from build123d import *

# Parameters (mm, degrees)
F0_R     = 35
F1_DEPTH = 6.5
F2_R     = 23.5
F3_DEPTH = 6.5
F4_R     = 32
F4_R_2   = 26
F5_DEPTH = 4
F7_DEPTH = 2
F8_R     = 6
F9_DEPTH = 4


with BuildPart() as f1:
    # F0 (on Top) → F1 (new body)
    with BuildSketch(Plane.XY):
        Circle(F0_R)
    extrude(amount=F1_DEPTH)

    # F2 (on face) → F3 (cut, through all)
    with BuildSketch(Plane.XY.offset(6.5)):
        Circle(F2_R)
    extrude(amount=-F3_DEPTH, mode=Mode.SUBTRACT)

    # F4 (on face) → F5 (cut)
    with BuildSketch(Plane(origin=(0, 0, 0), x_dir=(1, 0, 0), z_dir=(0, 0, -1))):
        Circle(F4_R)
        Circle(F4_R_2, mode=Mode.SUBTRACT)
    extrude(amount=-F5_DEPTH, mode=Mode.SUBTRACT)

    # F6 (on Top) → F7 (cut)
    with BuildSketch(Plane.XY):
        Polygon((-26, 5), (-26, -5), (-8.6602540378, -5), (-17.3301270189, -20.0166604984), (-8.6698729811, -25.0166604984), (0, -10), (8.6698729811, -25.0166604984), (17.3301270189, -20.0166604984), (8.6602540378, -5), (26, -5), (26, 5), (8.6602540378, 5), (17.3301270189, 20.0166604984), (8.6698729811, 25.0166604984), (0, 10), (-8.6698729811, 25.0166604984), (-17.3301270189, 20.0166604984), (-8.6602540378, 5), align=None)
    extrude(amount=F7_DEPTH, mode=Mode.SUBTRACT)

    # F8 (on Top) → F9 (join)
    with BuildSketch(Plane.XY):
        with Locations((0, -29.25)):
            Circle(F8_R)
        with Locations((25.3312430607, -14.625)):
            Circle(F8_R)
        with Locations((25.3312430607, 14.625)):
            Circle(F8_R)
        with Locations((0, 29.25)):
            Circle(F8_R)
        with Locations((-25.3312430607, 14.625)):
            Circle(F8_R)
        with Locations((-25.3312430607, -14.625)):
            Circle(F8_R)
    extrude(amount=F9_DEPTH)


solid = f1.part
Geometry check sheet. Reference: the model listing, model coordinates, mm. A direction names the side the tool comes from. Coordinates: 2 decimals unless noted, no trailing zeros. Order: outer loops, then holes, each group sorted by start corner. A loop starts at its lowest first (then second) coordinate and runs counter-clockwise, first axis right, second up. Notation, with made-up numbers: (21.5, 49) -> (67.5, 49) arc R24 cw to (67.5, 81) -> close; hole circle Ø5 at (64.25, 52). An arc over 180 degrees is marked (long way). Use a Markdown table: item, result. Add a question column.
1. Cross-section at A-A (x = 0). Enter the section's corners in (y, z), and give its area (4 significant figures).
2. Go/stop test with flat-tipped pins: pin 1 Ø2 at (x, y) = (-12, -19.5) entering from -Z; pin 2 Ø2 at (x, z) = (-24.5, 1.5) entering from -Y; pin 3 Ø0.5 at (x, y) = (-20, 11) entering from +Z; pin 4 Ø1.6 at (x, z) = (-24, 1) entering from +Y. Record where each tip stops, or that it passes through.
3. Material ranges on L1, parallel to X at y = 5.5, z = 3.25; L2, parallel to Y at x = 0, z = 2.5; L3, parallel to X at y = 1, z = 2.25, recorded low to high.
4. Mould release check, pull along X, two halves, no side actions. Record for faces 3 (the face through (-28, -21, 3)), 4 (the face through (5, -23.3, 0)), 5 (the face through (20.124, 11.644, 1.972)), 6 (the face through (-26, -0.1, 2.4)): pulls with the +X half, pulls with the -X half, needs draft (parallel to the pull), parting line crosses it, or undercut.
5. Cross-section at B-B (y = 0). Enter the section's corners in (x, z).
6. Set-up check for faces 1 (the face through (-13, -21, 2)), 2 (the face through (7, -23, 6.5)): record each of +Z, -Z, +X, -X, +Y, -Y from which the full face is reachable in a straight line by a thin tool's end or side.
Filled sheet:
| question | item | result |
|---|---|---|
| 1 | outline | (-35.25, 0) -> (-23.25, 0) -> (-23.25, 4) -> (-23.5, 4) -> (-23.5, 6.5) -> (-35, 6.5) -> (-35, 4) -> (-35.25, 4) -> close; (23.25, 0) -> (35.25, 0) -> (35.25, 4) -> (35, 4) -> (35, 6.5) -> (23.5, 6.5) -> (23.5, 4) -> (23.25, 4) -> close |
| 1 | area | 153.5 mm2 |
| 2 | pin 1 | z = 2 |
| 2 | pin 2 | y = -25.94 |
| 2 | pin 3 | through |
| 2 | pin 4 | y = 26.21 |
| 3 | L1 | -34.57 to -31.52, -25.41 to -22.85, 22.85 to 25.41, 31.52 to 34.57 |
| 3 | L2 | -35.25 to -23.25, 23.25 to 35.25 |
| 3 | L3 | -34.99 to -31.98, -25.98 to -23.48, 23.48 to 25.98, 31.98 to 34.99 |
| 4 | face 3 | parting line crosses it |
| 4 | face 4 | needs draft |
| 4 | face 5 | undercut |
| 4 | face 6 | undercut |
| 5 | outline | (-35, 0) -> (-32, 0) -> (-32, 4) -> (-26, 4) -> (-26, 2) -> (-23.5, 2) -> (-23.5, 6.5) -> (-35, 6.5) -> close; (23.5, 2) -> (26, 2) -> (26, 4) -> (32, 4) -> (32, 0) -> (35, 0) -> (35, 6.5) -> (23.5, 6.5) -> close |
| 6 | face 1 | -Z |
| 6 | face 2 | +Z, +X, -X, +Y, -Y |
